Part model, mm, in its own coordinate system. Face numbers are marked on the shaded views. A direction names the side the tool comes from. Round coordinates to 2 decimals unless told otherwise and drop trailing zeros. Loops run counter-clockwise (first coordinate to the right, second up) from the corner with the lowest first, then second, coordinate; pieces in that order, holes last. Notation, with made-up numbers: (69, -7) - (128, -7) arc R30 cw to (128, 30) - close; hole circle Ø3 at (-24, 34). An arc over 180 degrees is marked (long way). Put each result on its own line as item: value.
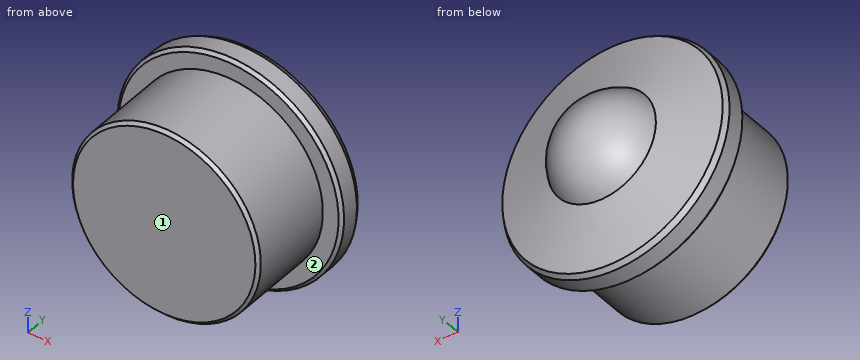
from build123d import *
from OCP.BRepFilletAPI import BRepFilletAPI_MakeChamfer

# Parameters (mm, degrees)
CHAMFER_1_SIZE  = 0.5
CHAMFER_1_SIZE2 = 0.70589663


with BuildPart() as part:
    # 草图2 → 旋转1 (revolve)
    with BuildSketch(Plane.XY, mode=Mode.PRIVATE) as revolve_1_sk:
        with BuildLine():
            Line((0, 0), (0, 26))
            ThreePointArc((0, 26), (5.117983001, 24.508173408), (8.63278634, 20.5))
            Line((8.63278634, 20.5), (18, 18))
            Line((18, 18), (18, 14))
            Line((18, 14), (15, 14))
            Line((15, 14), (15, 0))
            Line((15, 0), (0, 0))
        make_face()
    revolve(revolve_1_sk.sketch.rotate(Axis((0, 0, 0), (0, 1, 0)), 90), axis=Axis((0, 0, 0), (0, 1, 0)))

    # 倒角1: one chamfer whose edges measure the first distance from different faces: ONE call of the kernel's chamfer builder (chamfer() names one face for all edges)
    chamfer_1_edges_1 = [part.edges().sort_by_distance(p)[0] for p in [
        (0, 18, 18),
    ]]
    chamfer_1_side_1 = [part.faces().sort_by_distance(p)[0] for p in [
        (0, 19.25, 13.31639317),
    ]]
    chamfer_1_edges_2 = [part.edges().sort_by_distance(p)[0] for p in [
        (0, 14, 18),
        (0, 0, 15),
    ]]
    chamfer_1 = BRepFilletAPI_MakeChamfer(part.part.solid().wrapped)
    for e in chamfer_1_edges_1:
        chamfer_1.Add(CHAMFER_1_SIZE, CHAMFER_1_SIZE2, e.wrapped, chamfer_1_side_1[0].wrapped)  # the first distance lies on this face
    for e in chamfer_1_edges_2:
        chamfer_1.Add(CHAMFER_1_SIZE, e.wrapped)
    add(Compound.cast(chamfer_1.Shape()), mode=Mode.REPLACE)


solid = part.part
1. Band-saw the part on A-A (y = 9). List the corners of the cut face in (x, z), plus the area to 3 significant figures.
A:
outline: circle Ø30 at (0, 0)
area: 707 mm²
2. Tool access for the marked faces 1 and 2: list every direction of +Z, -Z, +X, -X, +Y, -Y with a clear straight run to the whole face (end or side of a thin tool).
A:
face 1: +Z, -Z, +X, -X, -Y
face 2: -Y
3. Probe line 1 along X through (y, z) = (12.5, 0); line 2 along X through (y, z) = (5.25, 6); line 3 along Z through (x, y) = (3, 5.5). List the from-to ranges inside material, lowest first. Write a range as [from, to].
A:
line 1: x = [-15, 15]
line 2: x = [-13.75, 13.75]
line 3: z = [-14.7, 14.7]
4. Pin check, flat tips, straight feed: P1, Ø5, axis at x = -6, z = -2.5, coming from the +Y side; P2, Ø1.5, axis at x = -13, y = 3, coming from the +Z side; P3, Ø3, axis at y = 14, z = -1, coming from the -X side; P4, Ø3, axis at y = 11, z = -7.5, coming from the -X side. Stop position of each tip, or through.
A:
P1: stops at y = 25.12
P2: stops at z = 8.66
P3: stops at x = -18
P4: stops at x = -13.75
5. Band-saw the part on B-B (y = 22.75). List the corners of the cut face in (x, z), plus the area to 3 significant figures.
A:
outline: circle Ø14.33 at (0, 0)
area: 161 mm²
